Autodesk Inventor part; units mm, degrees
ref_plane "YZ Plane" through (0, 0, 0) normal (1, 0, 0) x (0, 1, 0)
ref_plane "XZ Plane" through (0, 0, 0) normal (0, 1, 0) x (-1, 0, 0)
ref_plane "XY Plane" through (0, 0, 0) normal (0, 0, 1) x (1, 0, 0)
sketch "Sketch1" plane through (0, 0, 0) normal (0, 0, 1) x (1, 0, 0)
  line L0 (-12.6808, 7.3656) -> (0.0383, 14.6647)
  line L1 (0.0383, 14.6647) -> (12.7192, 7.2991)
  line L2 (12.7192, 7.2991) -> (12.6808, -7.3656)
  line L3 (12.6808, -7.3656) -> (-0.0383, -14.6647)
  line L4 (-0.0383, -14.6647) -> (-12.7192, -7.2991)
  line L5 (-12.7192, -7.2991) -> (-12.6808, 7.3656)
  point P0 (0, 0)
  dimension "d10" = 29.3294
extrude "Extrusion1" add sketch "Sketch1" along normal blind 149.255
sketch "Sketch2" plane through (0, 0, 0) normal (0, 0, -1) x (-1, 0, 0)
  circle A0 centre (0, 0) radius 10
  dimension "d13" = 20
sketch "Sketch3" plane through (0, 0, 149.255) normal (0, 0, 1) x (1, 0, 0)
  circle A0 centre (0, 0) radius 10
  dimension "d14" = 20
extrude "Extrusion2" add sketch "Sketch3" along normal blind 85
extrude "Extrusion3" add sketch "Sketch2" along normal blind 85
properties part number "HexBar1Inch"
Could you check a few things on this model? Use its own coordinates, in mm. A direction names the side the tool comes from. Give positions to 0.01 mm unless a question says otherwise; leave off trailing zeros. Loops run counter-clockwise (first coordinate to the right, second up) from the corner with the lowest first, then second, coordinate; pieces in that order, holes last. Notation, with made-up numbers: (28, 49) - (43, 49) arc R32 ccw to (43, 87) - close; hole circle Ø8 at (48, 29.25). An arc over 180 degrees is marked (long way). Answer in a Markdown table with one row per item. Add a question column.
Q1. If we section it at C-C (z = 7): List the corners of the cut face in (x, y) for me.
Q2. If we section it at B-B (x = 5.5): List the corners of the cut face in (y, z) for me (3 decimals), plus the area to 3 significant figures.
Q3. Which directions (+Z, -Z, +X, -X, +Y, -Y) give clear straight access to the entire face, cutting with the end or side of a thin tool? Please do faces 1 (the face through (2.17, 9.76, -41.9)), 2 (the face through (-2.17, 9.76, 191.16)), 3 (the face through (-6.29, -11.033, 73.583)).
Q4. For pin 1 (3 mm diameter, centred on x = -2.5, z = 123, fed in from -Y); pin 2 (4 mm diameter, centred on x = -1.5, z = 54.5, fed in from -Y); pin 3 (4 mm diameter, centred on x = -10, z = 110, fed in from -Y); pin 4 (1.5 mm diameter, centred on y = -8.5, z = 193, fed in from +X), each with a flat end and sliding along its axis, tell me the tip position at first contact or that it passes through.
Q5. If we section it at D-D (z = 182): List the corners of the cut face in (x, y) for me.
Q6. Please list where these lines run through material, in increasing order: L1, parallel to X at y = 2.25, z = 138; L2, parallel to Z at x = -5.75, y = -8.25 (3 decimals); L3, parallel to X at y = -1, z = 217.5. Write a range as from..to.
Q7. If we section it at A-A (y = 0): List the corners of the cut face in (x, z) for me (3 decimals).
The answers:
| question | item | result |
|---|---|---|
| 1 | outline | (-12.72, -7.3) - (-0.04, -14.66) - (12.68, -7.37) - (12.72, 7.3) - (0.04, 14.66) - (-12.68, 7.37) - close |
| 2 | outline | (-11.486, 0) - (-8.352, 0) - (-8.352, -85) - (8.352, -85) - (8.352, 0) - (11.492, 0) - (11.492, 149.255) - (8.352, 149.255) - (8.352, 234.255) - (-8.352, 234.255) - (-8.352, 149.255) - (-11.486, 149.255) - close |
| 2 | area | 6,270 mm^2 |
| 3 | face 1 | -Z |
| 3 | face 2 | +Z |
| 3 | face 3 | +Z, -Z, -X, -Y |
| 4 | pin 1 | stops at y = -14.11 |
| 4 | pin 2 | stops at y = -14.66 |
| 4 | pin 3 | stops at y = -10.04 |
| 4 | pin 4 | stops at x = 6.32 |
| 5 | outline | circle Ø20 at (0, 0) |
| 6 | L1 | x = -12.69..12.71 |
| 6 | L2 | z = 0..149.255 |
| 6 | L3 | x = -9.95..9.95 |
| 7 | outline | (-12.7, 0) - (-10, 0) - (-10, -85) - (10, -85) - (10, 0) - (12.7, 0) - (12.7, 149.255) - (10, 149.255) - (10, 234.255) - (-10, 234.255) - (-10, 149.255) - (-12.7, 149.255) - close |
